```python
from build123d import *

# Parameters (mm, degrees)
SKETCH3_W                         = 57.15
SKETCH3_H                         = 76.2
BOSS_EXTRUDE2_DEPTH               = 31.75
SKETCH4_W                         = 49.53
SKETCH4_H                         = 68.58
CUT_EXTRUDE2_DEPTH                = 26.67
POWER_HOLE_REACH                  = 102.402
SKETCH5_W                         = 9.398
SKETCH5_H                         = 11.43
MOTOR_MOUNTING_SHAPE_DEPTH        = 57.15
MOTOR_MOUNTING_HOLES_REACH        = 119.37
SKETCH8_R                         = 1.6
SKETCH7_W                         = 7.62
SKETCH7_H                         = 29.66
TRAY_SUPPORT_MOUNTING_SHAPE_DEPTH = 36.83
SKETCH9_W                         = 20.32
SKETCH9_H                         = 12.7
CUT_EXTRUDE3_DEPTH                = 16.51
SKETCH10_W                        = 6.35
SKETCH10_H                        = 46.54
CUT_EXTRUDE4_DEPTH                = 36.83
SKETCH11_R                        = 1.905
CUT_EXTRUDE5_DEPTH                = 97.497020291
BIGBUTTONWIREHOLE_REACH           = 104.123
SKETCH12_R                        = 1.905
BOSS_EXTRUDE3_DEPTH               = 20.32
FILLET2_R                         = 2.54
FILLET1_R                         = 2.54


with BuildPart() as part:
    # Sketch3 → Boss-Extrude2 (new body)
    with BuildSketch(Plane(origin=(0, 0, 0), x_dir=(-1, 0, 0), z_dir=(0, 1, 0))):
        with Locations((28.575, 38.1)):
            Rectangle(SKETCH3_W, SKETCH3_H)
    extrude(amount=-BOSS_EXTRUDE2_DEPTH)

    # Sketch4 → Cut-Extrude2 (cut)
    with BuildSketch(Plane.XZ.offset(31.75)):
        with Locations((-28.575, 38.1)):
            Rectangle(SKETCH4_W, SKETCH4_H)
    extrude(amount=-CUT_EXTRUDE2_DEPTH, mode=Mode.SUBTRACT)

    # Sketch5 → Power Hole (cut, up to next)
    with BuildSketch(Plane(origin=(-57.15, 0, 0), x_dir=(0, 0, -1), z_dir=(1, 0, 0)), mode=Mode.PRIVATE) as power_hole_sk1:
        with Locations((-9.779, -22.225)):
            Rectangle(SKETCH5_W, SKETCH5_H)
    power_hole_tool1 = extrude(power_hole_sk1.sketch, amount=POWER_HOLE_REACH, mode=Mode.PRIVATE) & part.part
    add(power_hole_tool1.solids().sort_by_distance((-57.15, -22.225, 9.779))[0], mode=Mode.SUBTRACT)

    # Sketch6 → Motor Mounting Shape (add)
    with BuildSketch(Plane.ZY.offset(57.15)):
        Polygon((46.54, 0), (46.54, 36.83), (0, 36.83), (0, 34.29), (44, 34.29), (44, 0), align=None)
    extrude(amount=-MOTOR_MOUNTING_SHAPE_DEPTH)

    # Sketch8 → Motor-Mounting-Holes (cut, up to next)
    with BuildSketch(Plane(origin=(0, 36.83, 0), x_dir=(1, 0, 0), z_dir=(0, 1, 0)), mode=Mode.PRIVATE) as motor_mounting_holes_sk1:
        with Locations(Location((-44.075, -7.77, 0), (0, 0, 270))):
            Circle(SKETCH8_R)
    motor_mounting_holes_tool1 = extrude(motor_mounting_holes_sk1.sketch, amount=-MOTOR_MOUNTING_HOLES_REACH, mode=Mode.PRIVATE) & part.part
    # Sketch8 → Motor-Mounting-Holes (cut, up to next)
    with BuildSketch(Plane(origin=(0, 36.83, 0), x_dir=(1, 0, 0), z_dir=(0, 1, 0)), mode=Mode.PRIVATE) as motor_mounting_holes_sk2:
        with Locations(Location((-13.075, -7.77, 0), (0, 0, 270))):
            Circle(SKETCH8_R)
    motor_mounting_holes_tool2 = extrude(motor_mounting_holes_sk2.sketch, amount=-MOTOR_MOUNTING_HOLES_REACH, mode=Mode.PRIVATE) & part.part
    # Sketch8 → Motor-Mounting-Holes (cut, up to next)
    with BuildSketch(Plane(origin=(0, 36.83, 0), x_dir=(1, 0, 0), z_dir=(0, 1, 0)), mode=Mode.PRIVATE) as motor_mounting_holes_sk3:
        with Locations(Location((-13.075, -38.77, 0), (0, 0, 270))):
            Circle(SKETCH8_R)
    motor_mounting_holes_tool3 = extrude(motor_mounting_holes_sk3.sketch, amount=-MOTOR_MOUNTING_HOLES_REACH, mode=Mode.PRIVATE) & part.part
    # Sketch8 → Motor-Mounting-Holes (cut, up to next)
    with BuildSketch(Plane(origin=(0, 36.83, 0), x_dir=(1, 0, 0), z_dir=(0, 1, 0)), mode=Mode.PRIVATE) as motor_mounting_holes_sk4:
        with Locations(Location((-44.075, -38.77, 0), (0, 0, 270))):
            Circle(SKETCH8_R)
    motor_mounting_holes_tool4 = extrude(motor_mounting_holes_sk4.sketch, amount=-MOTOR_MOUNTING_HOLES_REACH, mode=Mode.PRIVATE) & part.part
    # Sketch8 → Motor-Mounting-Holes (cut, up to next)
    with BuildSketch(Plane(origin=(0, 36.83, 0), x_dir=(1, 0, 0), z_dir=(0, 1, 0)), mode=Mode.PRIVATE) as motor_mounting_holes_sk5:
        with BuildLine():
            Line((-37.465, 0), (-19.685, 0))
            Line((-19.685, 0), (-19.685, -23.27))
            ThreePointArc((-19.685, -23.27), (-28.575, -32.16), (-37.465, -23.27))
            Line((-37.465, -23.27), (-37.465, 0))
        make_face()
    motor_mounting_holes_tool5 = extrude(motor_mounting_holes_sk5.sketch, amount=-MOTOR_MOUNTING_HOLES_REACH, mode=Mode.PRIVATE) & part.part
    add(motor_mounting_holes_tool1.solids().sort_by_distance((-44.075, 36.83, 7.77))[0], mode=Mode.SUBTRACT)
    add(motor_mounting_holes_tool2.solids().sort_by_distance((-13.075, 36.83, 7.77))[0], mode=Mode.SUBTRACT)
    add(motor_mounting_holes_tool3.solids().sort_by_distance((-13.075, 36.83, 38.77))[0], mode=Mode.SUBTRACT)
    add(motor_mounting_holes_tool4.solids().sort_by_distance((-44.075, 36.83, 38.77))[0], mode=Mode.SUBTRACT)
    add(motor_mounting_holes_tool5.solids().sort_by_distance((-28.575, 36.83, 15.191166))[0], mode=Mode.SUBTRACT)

    # Sketch7 → Tray Support Mounting Shape (add)
    with BuildSketch(Plane(origin=(0, 0, 0), x_dir=(1, 0, 0), z_dir=(0, 1, 0))):
        with Locations((-42.545, -61.37)):
            Rectangle(SKETCH7_W, SKETCH7_H)
        with Locations((-14.605, -61.37)):
            Rectangle(SKETCH7_W, SKETCH7_H)
    extrude(amount=TRAY_SUPPORT_MOUNTING_SHAPE_DEPTH)

    # Sketch9 → Cut-Extrude3 (cut)
    with BuildSketch(Plane.XZ.offset(5.08)):
        with Locations((-28.575, 45.27)):
            Rectangle(SKETCH9_W, SKETCH9_H)
    extrude(amount=-CUT_EXTRUDE3_DEPTH, mode=Mode.SUBTRACT)

    # Sketch10 → Cut-Extrude4 (cut)
    with BuildSketch(Plane(origin=(0, 36.83, 0), x_dir=(1, 0, 0), z_dir=(0, 1, 0))):
        with Locations((-53.975, -23.27)):
            Rectangle(SKETCH10_W, SKETCH10_H)
        with Locations((-3.175, -23.27)):
            Rectangle(SKETCH10_W, SKETCH10_H)
    extrude(amount=-CUT_EXTRUDE4_DEPTH, mode=Mode.SUBTRACT)

    # Sketch11 → Cut-Extrude5 (cut, through all)
    with BuildSketch(Plane.ZY.offset(46.355)):
        with Locations((61.37, 24.13)):
            Circle(SKETCH11_R)
        with Locations((61.37, 12.7)):
            Circle(SKETCH11_R)
    extrude(amount=-CUT_EXTRUDE5_DEPTH, mode=Mode.SUBTRACT)

    # Sketch12 → BigButtonWireHole (cut, up to next)
    with BuildSketch(Plane(origin=(0, 0, 0), x_dir=(0, 0, -1), z_dir=(1, 0, 0)), mode=Mode.PRIVATE) as bigbuttonwirehole_sk1:
        with Locations((-67.31, -22.86)):
            Circle(SKETCH12_R)
    bigbuttonwirehole_tool1 = extrude(bigbuttonwirehole_sk1.sketch, amount=-BIGBUTTONWIREHOLE_REACH, mode=Mode.PRIVATE) & part.part
    add(bigbuttonwirehole_tool1.solids().sort_by_distance((0, -22.86, 67.31))[0], mode=Mode.SUBTRACT)

    # Sketch13 → Boss-Extrude3 (add)
    with BuildSketch(Plane(origin=(-38.735, 0, 0), x_dir=(0, 0, -1), z_dir=(1, 0, 0))):
        with BuildLine():
            Line((-46.54, 11.43), (-46.54, 15.24))
            ThreePointArc((-46.54, 15.24), (-52.826179285, 12.636179285), (-55.43, 6.35))
            Line((-55.43, 6.35), (-55.43, 0))
            Line((-55.43, 0), (-51.62, 0))
            Line((-51.62, 0), (-51.62, 6.35))
            ThreePointArc((-51.62, 6.35), (-50.132102448, 9.942102448), (-46.54, 11.43))
        make_face()
    extrude(amount=BOSS_EXTRUDE3_DEPTH)

    # Fillet2
    fillet2_edges = [part.edges().sort_by_distance(p)[0] for p in [
        (-18.415, 5.715, 44),
        (-38.735, 5.715, 44),
        (-28.575, 0, 38.92),
        (-18.415, 0.635, 51.62),
        (-38.735, 0.635, 51.62),
        (-28.575, 11.43, 44),
        (-38.735, -5.08, 45.27),
        (-28.575, -5.08, 38.92),
        (-18.415, -5.08, 45.27),
        (-28.575, -5.08, 51.62),
        (-38.735, 9.942102448, 50.132102448),
        (-18.415, 9.942102448, 50.132102448),
        (-38.735, 0, 41.46),
        (-18.415, 0, 41.46),
    ]]
    fillet(fillet2_edges, radius=FILLET2_R - 0.0001)  # a hair under: the kernel refuses the full size

    # Fillet1
    fillet1_edges = [part.edges().sort_by_distance(p)[0] for p in [
        (-38.735, 26.035, 46.54),
        (-42.545, 36.83, 76.2),
        (-38.735, 36.83, 61.37),
        (-18.415, 26.035, 46.54),
        (-18.415, 36.83, 61.37),
        (-14.605, 36.83, 76.2),
        (-57.15, -31.75, 38.1),
        (-28.575, -31.75, 76.2),
        (-50.8, 35.56, 0),
        (-6.35, 35.56, 0),
        (-28.575, 15.24, 46.54),
        (0, -31.75, 38.1),
        (-57.15, 0, 38.1),
        (-28.575, 0, 0),
        (0, 0, 38.1),
        (0, -15.875, 76.2),
        (-57.15, -15.875, 76.2),
        (-19.685, 35.56, 0),
        (-37.465, 35.56, 0),
        (-57.15, -15.875, 0),
        (0, -15.875, 0),
        (-28.575, -31.75, 0),
        (-28.575, 36.83, 46.54),
    ]]
    fillet(fillet1_edges, radius=FILLET1_R)


solid = part.part
```
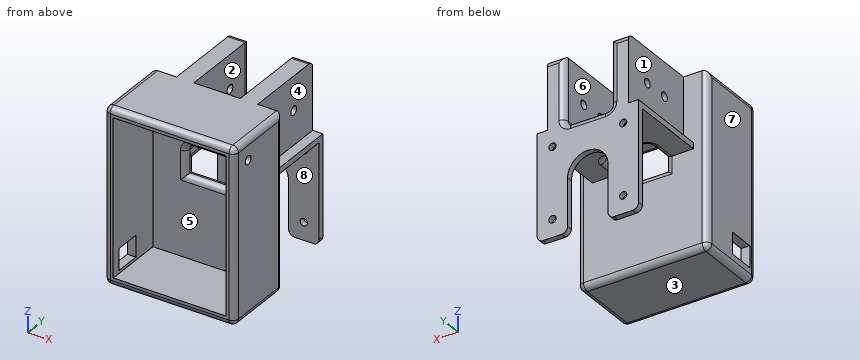
Can you work these out from the model? Positions are in its coordinate system, mm. Face numbers are marked on the shaded views. A direction names the side the tool comes from. Give positions to 0.01 mm unless a question says otherwise; leave off trailing zeros. Loops run counter-clockwise (first coordinate to the right, second up) from the corner with the lowest first, then second, coordinate; pieces in that order, holes last. Notation, with made-up numbers: M 21,42 L 80,42 A36 cw 80,81 Z; hole C 3,17 d8. An arc over 180 degrees is marked long. Use one line per item in the form item = value. Start each with the question number.
(1) I want a section at A-A, the plane y = 24.13. Write out the boundary of the cut face in (x, z) (3 decimals).
(2) On a 3-axis mill with a long thin cutter (end or side, diameter ignored), from which of +Z, -Z, +X, -X, +Y, -Y can I reach the whole of each face in a straight line? I mean the marked faces 4, 5, 6, 7 and 8. Say none if no direction works.
(3) Thinking about a two-plate mould opening in X: for the marked faces 1, 2 and 3, which applies, released by +X, released by -X, zero draft, split by the parting line, or undercut?
(4) I'm going to push flat-ended pins straight in: P1, Ø5, axis at y = 5, z = 46, coming from the +X side; P2, Ø10, axis at x = -25.5, z = 61, coming from the +Y side; P3, Ø4, axis at y = 8.5, z = 42.5, coming from the +X side. Where does each tip first touch, or does it pass through?
(5) Please list where these lines run through material, in increasing order: line 1 (X direction, y = 35.9, z = 38.77) (3 decimals); line 2 (X direction, y = 35.6, z = 7.77) (3 decimals); line 3 (Y direction, x = -43.5, z = 14).
(6) I want a section at C-C, the plane z = 62. State how many separate pieces and enclosed holes the cut face has, and give its area (3 significant figures).
Worked out:
q1.outline = M -50.8,44 L -6.35,44 L -6.35,46.54 L -10.795,46.54 L -10.795,59.465 L -18.415,59.465 L -18.415,49.08 A2.54 cw -20.955,46.54 L -36.195,46.54 A2.54 cw -38.735,49.08 L -38.735,59.465 L -46.355,59.465 L -46.355,46.54 L -50.8,46.54 Z; M -46.355,63.275 L -38.735,63.275 L -38.735,76.2 L -46.355,76.2 Z; M -18.415,63.275 L -10.795,63.275 L -10.795,76.2 L -18.415,76.2 Z
q2.face_4 = +Z, +X, +Y
q2.face_5 = -Y
q2.face_6 = +Z, +Y
q2.face_7 = +Z, -Z, -X, +Y, -Y
q2.face_8 = -Z, +X, -X
q3.face_1 = released by -X
q3.face_2 = undercut
q3.face_3 = zero draft
q4.P1 = -6.35
q4.P2 = 0
q4.P3 = -6.35
q5.line_1 = -50.8 to -45.675, -42.475 to -14.675, -11.475 to -6.35
q5.line_2 = -50.8 to -45.675, -42.475 to -37.465, -19.685 to -14.675, -11.475 to -6.35
q5.line_3 = -5.08 to 0, 34.29 to 36.83
q6.separate_pieces = 5
q6.enclosed_holes = 0
q6.area = 937 mm²
